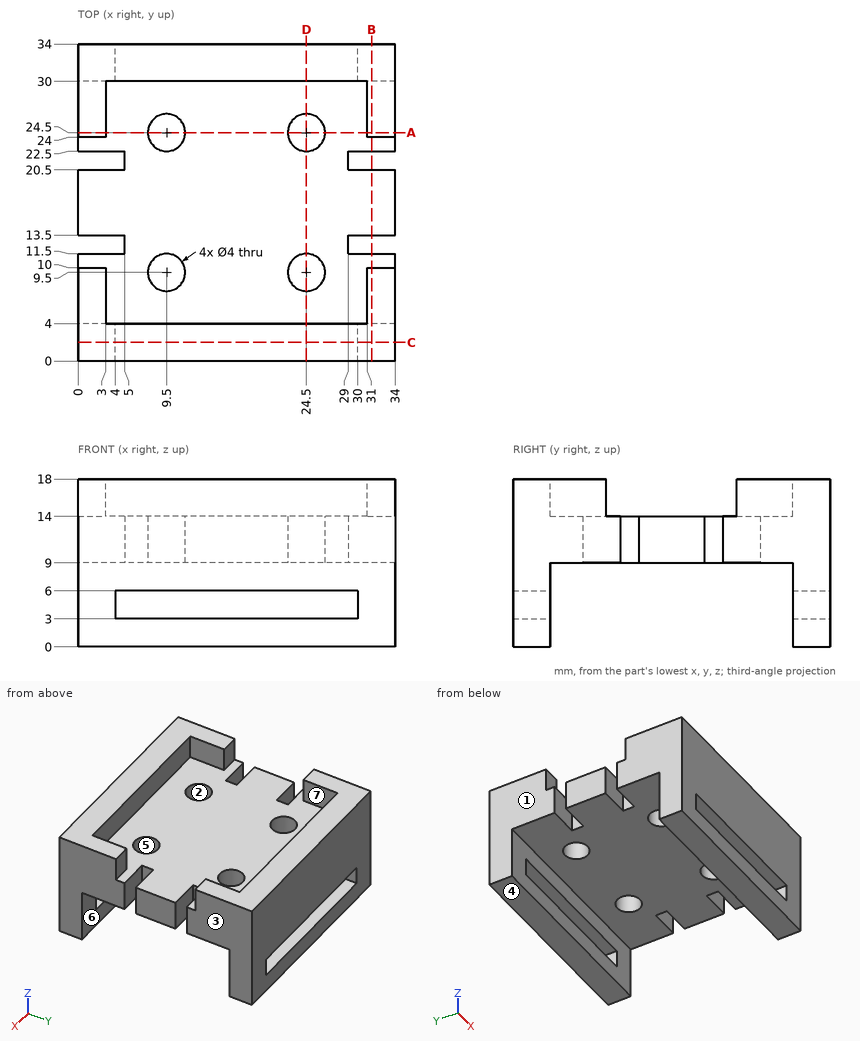
The figure shows three views and two pictorial views of one solid part (mm, origin at its lowest corner). Answer the questions. A direction names the side the tool comes from. Coordinates: 2 decimals unless noted, no trailing zeros. Write each loop counter-clockwise with the first axis right and the second up, starting at its lowest first coordinate (ties: lowest second). Pieces come first, ordered by that corner, then holes.
1. For a pull along X with two mould halves and no side action, classify the marked faces 1, 2, 3 and 4 as +X half, -X half, draft (parallel to the pull), parting line (faces both ways), or undercut.
Results list:
face 1: -X half
face 2: undercut
face 3: +X half
face 4: draft
2. The part is cut by section D-D, the plane x = 24.5. Write down the section's boundary in (y, z).
Results list:
outline: (0, 0) - (4, 0) - (4, 3) - (0, 3) - close; (0, 6) - (4, 6) - (4, 9) - (7.5, 9) - (7.5, 14) - (4, 14) - (4, 18) - (0, 18) - close; (11.5, 9) - (22.5, 9) - (22.5, 14) - (11.5, 14) - close; (26.5, 9) - (30, 9) - (30, 6) - (34, 6) - (34, 18) - (30, 18) - (30, 14) - (26.5, 14) - close; (30, 0) - (34, 0) - (34, 3) - (30, 3) - close
3. The part is cut by section A-A, the plane y = 24.5. Write down the section's boundary in (x, z).
Results list:
outline: (0, 9) - (7.5, 9) - (7.5, 14) - (3, 14) - (3, 18) - (0, 18) - close; (11.5, 9) - (22.5, 9) - (22.5, 14) - (11.5, 14) - close; (26.5, 9) - (34, 9) - (34, 18) - (31, 18) - (31, 14) - (26.5, 14) - close
4. The part is cut by section B-B, the plane x = 31.5. Write down the section's boundary in (y, z).
Results list:
outline: (0, 0) - (4, 0) - (4, 9) - (11.5, 9) - (11.5, 14) - (10, 14) - (10, 18) - (0, 18) - close; (13.5, 9) - (20.5, 9) - (20.5, 14) - (13.5, 14) - close; (22.5, 9) - (30, 9) - (30, 0) - (34, 0) - (34, 18) - (24, 18) - (24, 14) - (22.5, 14) - close
5. Flat-ended cylindrical pins translate along their axes: pin 1 (13 mm diameter, centred on x = 23, y = 14.5, fed in from -Z); pin 2 (8 mm diameter, centred on x = 21, y = 17, fed in from +Z). Find the tip coordinate at first contact, or state that the pin passes through.
Results list:
pin 1: stops at z = 9
pin 2: stops at z = 14
6. For the marked faces 5, 6 and 7, determine the directions among +Z, -Z, +X, -X, +Y, -Y from which every point of the face is accessible in a straight line to the end or side of a thin tool.
Results list:
face 5: +Z, -Z
face 6: -Z, +X, -X
face 7: +Z
7. Consider line 1 along Y through (x, z) = (24.5, 11.2); line 2 along Y through (x, z) = (14, 15.25); line 3 along X through (y, z) = (7, 16.5). Determine where each line is inside the solid, lowest interval first.
Results list:
line 1: y = 0 to 7.5, 11.5 to 22.5, 26.5 to 34
line 2: y = 0 to 4, 30 to 34
line 3: x = 0 to 3, 31 to 34
8. The part is cut by section C-C, the plane y = 2. Write down the section's boundary in (x, z), and give its area (3 significant figures).
Results list:
outline: (0, 0) - (34, 0) - (34, 18) - (0, 18) - close; hole (4, 3) - (30, 3) - (30, 6) - (4, 6) - close
area: 534 mm2
